from build123d import *

# Parameters (mm, degrees)
BOSS_EXTRUDE1_DEPTH = 23.8125
SKETCH2_R           = 2.5796875
CUT_EXTRUDE1_DEPTH  = 7.604
SKETCH3_R           = 4.7625
CUT_EXTRUDE2_DEPTH  = 7.604


with BuildPart() as part:
    # Sketch1 → Boss-Extrude1 (new body, symmetric)
    with BuildSketch(Plane.XY):
        with BuildLine():
            Line((0, -9.525), (0, 9.525))
            Line((0, 9.525), (-3.175, 9.525))
            Line((-3.175, 9.525), (-3.175, 4.064))
            ThreePointArc((-3.175, 4.064), (-4.445, 2.794), (-5.715, 4.064))
            Line((-5.715, 4.064), (-6.604, 4.064))
            Line((-6.604, 4.064), (-6.604, -4.064))
            Line((-6.604, -4.064), (-5.715, -4.064))
            ThreePointArc((-5.715, -4.064), (-4.445, -2.794), (-3.175, -4.064))
            Line((-3.175, -4.064), (-3.175, -9.525))
            Line((-3.175, -9.525), (0, -9.525))
        make_face()
    extrude(amount=BOSS_EXTRUDE1_DEPTH, both=True)

    # Sketch2 → Cut-Extrude1 (cut, through all)
    with BuildSketch(Plane.ZY.offset(6.604)):
        with Locations((16.2814, 0)):
            Circle(SKETCH2_R)
        with Locations((-16.2814, 0)):
            Circle(SKETCH2_R)
        Circle(SKETCH2_R)
    extrude(amount=-CUT_EXTRUDE1_DEPTH, mode=Mode.SUBTRACT)

    # Sketch3 → Cut-Extrude2 (cut, through all)
    with BuildSketch(Plane.ZY.offset(6.604)):
        with Locations((-16.2814, 0)):
            Circle(SKETCH3_R)
        with Locations((16.2814, 0)):
            Circle(SKETCH3_R)
    extrude(amount=-CUT_EXTRUDE2_DEPTH, mode=Mode.SUBTRACT)


solid = part.part
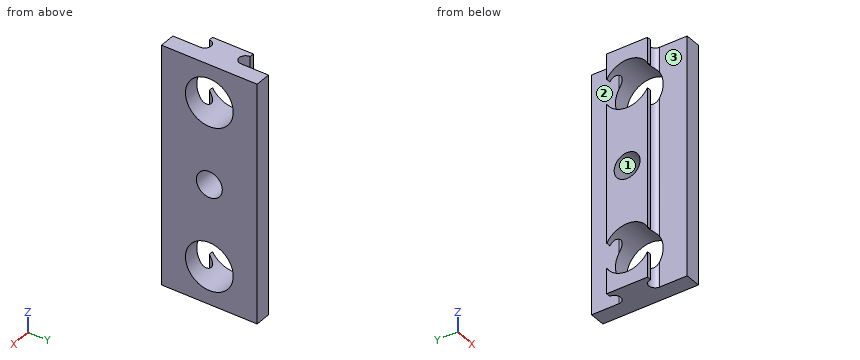
Could you check a few things on this model? Use its own coordinates, in mm. Face numbers are marked on the shaded views. A direction names the side the tool comes from. Coordinates: 2 decimals unless noted, no trailing zeros. Order: outer loops, then holes, each group sorted by start corner. A loop starts at its lowest first (then second) coordinate and runs counter-clockwise, first axis right, second up. Notation, with made-up numbers: (-13, 58) -> (37, 58) arc R21 cw to (37, 72) -> close; hole circle Ø8 at (35.25, -33.5). An arc over 180 degrees is marked (long way). One line per question, with ' | ' between items.
Q1. If I drill on L1, parallel to Z at x = -2.25, y = -0.25; L2, parallel to X at y = 6, z = -7.5 (3 decimals); L3, parallel to Z at x = -1.75, y = -2, over which ranges is the centre line in solid material (lowest first)?
Return value:
L1: -23.81 to -21.04, -11.53 to -2.57, 2.57 to 11.53, 21.04 to 23.81 | L2: -3.175 to 0 | L3: -23.81 to -20.6, -11.96 to -1.63, 1.63 to 11.96, 20.6 to 23.81
Q2. Imagine slicing it at C-C on y = 1.75. Please give me the cut outline in (x, z), and give its area (3 significant figures).
Return value:
outline: (-6.6, -23.81) -> (0, -23.81) -> (0, -20.71) -> (-6.6, -20.71) -> close; (-6.6, -11.85) -> (0, -11.85) -> (0, -1.9) -> (-6.6, -1.9) -> close; (-6.6, 1.9) -> (0, 1.9) -> (0, 11.85) -> (-6.6, 11.85) -> close; (-6.6, 20.71) -> (0, 20.71) -> (0, 23.81) -> (-6.6, 23.81) -> close | area: 172 mm²
Q3. On a 3-axis mill with a long thin cutter (end or side, diameter ignored), from which of +Z, -Z, +X, -X, +Y, -Y can I reach the whole of each face in a straight line? I mean the marked faces 1, 2 and 3. Say none if no direction works.
Return value:
face 1: +X, -X | face 2: +Z, -Z, -X, +Y | face 3: +Z, -Z, -X, -Y
Q4. Imagine slicing it at A-A on z = 0. Please give me the cut outline in (x, y) (3 decimals), and give its area (3 significant figures).
Return value:
outline: (-6.604, -4.064) -> (-5.715, -4.064) arc R1.27 cw to (-3.175, -4.064) -> (-3.175, -9.525) -> (0, -9.525) -> (0, -2.58) -> (-6.604, -2.58) -> close; (-6.604, 2.58) -> (0, 2.58) -> (0, 9.525) -> (-3.175, 9.525) -> (-3.175, 4.064) arc R1.27 cw to (-5.715, 4.064) -> (-6.604, 4.064) -> close | area: 49.2 mm²
Q5. Imagine slicing it at D-D on z = 12.5. Please give me the cut outline in (x, y) (3 decimals).
Return value:
outline: (-6.604, -4.064) -> (-5.715, -4.064) arc R1.27 cw to (-4.942, -2.895) -> (-6.604, -2.895) -> close; (-6.604, 2.895) -> (-4.942, 2.895) arc R1.27 cw to (-5.715, 4.064) -> (-6.604, 4.064) -> close; (-3.948, -2.895) arc R1.27 cw to (-3.175, -4.064) -> (-3.175, -9.525) -> (0, -9.525) -> (0, -2.895) -> close; (-3.948, 2.895) -> (0, 2.895) -> (0, 9.525) -> (-3.175, 9.525) -> (-3.175, 4.064) arc R1.27 cw to start
Q6. Imagine slicing it at B-B on x = -4.75. Please give me the cut outline in (y, z) (1 decimal), and give its area (3 significant figures).
Return value:
outline: (-2.8, -23.8) -> (2.8, -23.8) -> (2.8, -20.1) arc R4.8 cw to (-2.8, -20.1) -> close; (-2.8, -12.5) arc R4.8 cw to (2.8, -12.5) -> (2.8, 12.5) arc R4.8 cw to (-2.8, 12.5) -> close; (-2.8, 20.1) arc R4.8 cw to (2.8, 20.1) -> (2.8, 23.8) -> (-2.8, 23.8) -> close; hole circle Ø5.2 at (0, 0) | area: 148 mm²
Q7. I'm going to push flat-ended pins straight in: P1, Ø1, axis at x = -6, z = 21, coming from the -Y side; P2, Ø1.6, axis at y = -6.5, z = -3.5, coming from the -X side (3 decimals). Where does each tip first touch, or does it pass through?
Return value:
P1: y = -4.06 | P2: x = -3.175
